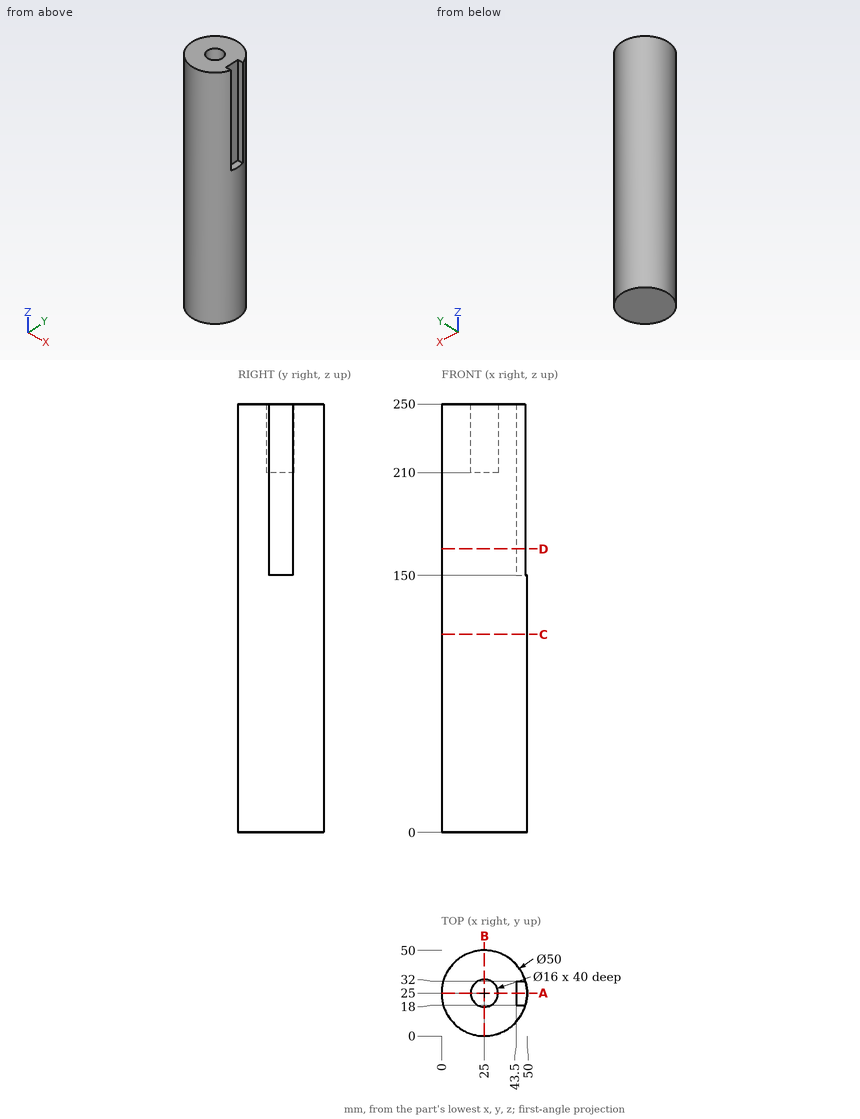
Study the drawing (mm; zero at the part's minimum x, y, z) and answer. Coordinates: 2 decimals unless noted, no trailing zeros. Loops run counter-clockwise (first coordinate to the right, second up) from the corner with the lowest first, then second, coordinate; pieces in that order, holes last. Notation, with made-up numbers: (24, -10) -> (46, -10) arc R8 cw to (46, -4) -> close; hole circle Ø11 at (84.25, 2.25). An arc over 180 degrees is marked (long way). Answer in a Markdown table with one row per item. Add a question column.
1. The part is cut by section A-A, the plane y = 25. Write down the section's boundary in (x, z), then the cut area to 3 significant figures.
2. The part is cut by section B-B, the plane x = 25. Write down the section's boundary in (y, z), then the cut area to 3 significant figures.
3. The part is cut by section C-C, the plane z = 115.5. Write down the section's boundary in (x, y).
4. The part is cut by section D-D, the plane z = 165.5. Write down the section's boundary in (x, y), then the cut area to 3 significant figures.
5. Flat-ended cylindrical pins translate along their axes: P1, Ø4.5, axis at x = 47, z = 187.5, coming from the +Y side; P2, Ø2, axis at y = 39.5, z = 119.5, coming from the -X side; P3, Ø7, axis at x = 48, y = 25, coming from the +Z side. Find the tip coordinate at first contact, or state that the pin passes through.
6. Consider line 1 (Y direction, x = 25, z = 224); line 2 (Z direction, x = 24.5, y = 19.5); line 3 (Y direction, x = 45.5, z = 232). Determine where each line is inside the solid, lowest interval first. Write a range as [from, to].
Answer below:
| question | item | result |
|---|---|---|
| 1 | outline | (0, 0) -> (50, 0) -> (50, 150) -> (43.5, 150) -> (43.5, 250) -> (33, 250) -> (33, 210) -> (17, 210) -> (17, 250) -> (0, 250) -> close |
| 1 | area | 11,200 mm2 |
| 2 | outline | (0, 0) -> (50, 0) -> (50, 250) -> (33, 250) -> (33, 210) -> (17, 210) -> (17, 250) -> (0, 250) -> close |
| 2 | area | 11,900 mm2 |
| 3 | outline | circle Ø50 at (25, 25) |
| 4 | outline | (43.5, 18) -> (43.5, 32) -> (49, 32) arc R25 ccw (long way) to (49, 18) -> close |
| 4 | area | 1,880 mm2 |
| 5 | P1 | y = 40.33 |
| 5 | P2 | x = 3.96 |
| 5 | P3 | z = 150 |
| 6 | line 1 | [0, 17], [33, 50] |
| 6 | line 2 | [0, 210] |
| 6 | line 3 | [10.69, 18], [32, 39.31] |
